Verification items for the finished model (mm, model axes). Face numbers are marked on the shaded views. A direction names the side the tool comes from. Coordinates: 2 decimals unless noted, no trailing zeros. Loops run counter-clockwise (first coordinate to the right, second up) from the corner with the lowest first, then second, coordinate; pieces in that order, holes last. Notation, with made-up numbers: (60.5, 18) -> (100.5, 18) arc R34 ccw to (100.5, 55) -> close; hole circle Ø5 at (-39.5, -15). An arc over 180 degrees is marked (long way). Answer as a JSON object with one key per item and string values. Group by question number.
Q1. Cross-section at B-B on z = -21.75. Record the boundary of the cut face in (x, y), and give its area (4 significant figures).
Q2. Cross-section at A-A on x = 0. Record the boundary of the cut face in (y, z), and give its area (3 significant figures).
Q3. Release check for a two-part mould opening along Z. For the marked faces 4 and 5 record: released by +Z, released by -Z, zero draft, split by the parting line, or undercut.
Q4. Cross-section at D-D on z = -4. Record the boundary of the cut face in (x, y), and give its area (3 significant figures).
Q5. Gauge pin test, flat ends, axial feed: pin 1 Ø1.5 at (y, z) = (3, 2.5) entering from +X; pin 2 Ø2 at (x, y) = (-1.5, 3.5) entering from -Z; pin 3 Ø1.5 at (x, y) = (1.5, 3) entering from +Z. Record the tip position at first contact, or that the pin passes through.
Q6. Cross-section at C-C on y = 3.7. Record the boundary of the cut face in (x, z).
Q7. Scan lines: L1, parallel to Z at x = 0, y = 4; L2, parallel to X at y = 4.25, z = -21.75; L3, parallel to Z at x = -1, y = 1.05. Record each from-to range of solid material in increasing order.
Q8. Set-up check for the marked faces 1, 2 and 3: record each of +Z, -Z, +X, -X, +Y, -Y from which the full face is reachable in a straight line by a thin tool's end or side.
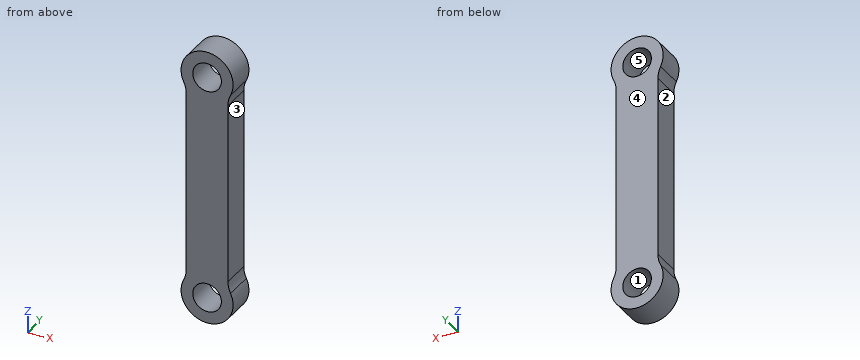
```python
from build123d import *

# Parameters (mm, degrees)
BOSS_EXTRUDE1_DEPTH = 5.5
SKETCH2_R           = 2.75
CUT_EXTRUDE2_DEPTH  = 6.5
SKETCH3_R           = 5
SKETCH3_R_2         = 2.75
BOSS_EXTRUDE2_DEPTH = 5.5
FILLET1_R           = 5


with BuildPart() as part:
    # Sketch1 → Boss-Extrude1 (new body)
    with BuildSketch(Plane(origin=(0, 0, 0), x_dir=(1, 0, 0), z_dir=(0, 1, 0))):
        with BuildLine():
            Line((-4, -21.75), (-4, 21.75))
            ThreePointArc((-4, 21.75), (0, 25.75), (4, 21.75))
            Line((4, 21.75), (4, -21.75))
            ThreePointArc((4, -21.75), (0, -25.75), (-4, -21.75))
        make_face()
    extrude(amount=BOSS_EXTRUDE1_DEPTH)

    # Sketch2 → Cut-Extrude2 (cut, through all)
    with BuildSketch(Plane(origin=(0, 5.5, 0), x_dir=(1, 0, 0), z_dir=(0, 1, 0))):
        with Locations((0, 21.75)):
            Circle(SKETCH2_R)
        with Locations((0, -21.75)):
            Circle(SKETCH2_R)
    extrude(amount=-CUT_EXTRUDE2_DEPTH, mode=Mode.SUBTRACT)

    # Sketch3 → Boss-Extrude2 (add)
    with BuildSketch(Plane(origin=(0, 5.5, 0), x_dir=(1, 0, 0), z_dir=(0, 1, 0))):
        with Locations((0, 21.75)):
            Circle(SKETCH3_R)
        with Locations((0, 21.75)):
            Circle(SKETCH3_R_2, mode=Mode.SUBTRACT)
        with Locations((0, -21.75)):
            Circle(SKETCH3_R)
        with Locations((0, -21.75)):
            Circle(SKETCH3_R_2, mode=Mode.SUBTRACT)
    extrude(amount=-BOSS_EXTRUDE2_DEPTH)

    # Fillet1
    fillet1_edges = [part.edges().sort_by_distance(p)[0] for p in [
        (-4, 2.75, -18.75),
        (4, 2.75, -18.75),
        (-4, 2.75, 18.75),
        (4, 2.75, 18.75),
    ]]
    fillet(fillet1_edges, radius=FILLET1_R)


solid = part.part
```
Computed values:
{
 "1": {"outline": "(-5, 0) -> (-2.75, 0) -> (-2.75, 5.5) -> (-5, 5.5) -> close; (2.75, 0) -> (5, 0) -> (5, 5.5) -> (2.75, 5.5) -> close", "area": "24.75 mm²"},
 "2": {"outline": "(0, -26.75) -> (5.5, -26.75) -> (5.5, -24.5) -> (0, -24.5) -> close; (0, -19) -> (5.5, -19) -> (5.5, 19) -> (0, 19) -> close; (0, 24.5) -> (5.5, 24.5) -> (5.5, 26.75) -> (0, 26.75) -> close", "area": "234 mm²"},
 "3": {"face 4": "zero draft", "face 5": "undercut"},
 "4": {"outline": "(-4, 0) -> (4, 0) -> (4, 5.5) -> (-4, 5.5) -> close", "area": "44.0 mm²"},
 "5": {"pin 1": "stops at x = 4", "pin 2": "stops at z = -26.72", "pin 3": "stops at z = 26.69"},
 "6": {"outline": "(-4.5, -19.57) arc R5 ccw (long way) to (4.5, -19.57) arc R5 cw to (4, -17.39) -> (4, 17.39) arc R5 cw to (4.5, 19.57) arc R5 ccw (long way) to (-4.5, 19.57) arc R5 cw to (-4, 17.39) -> (-4, -17.39) arc R5 cw to start; hole circle Ø5.5 at (0, -21.75); hole circle Ø5.5 at (0, 21.75)"},
 "7": {"L1": "z = -26.75 to -24.5, -19 to 19, 24.5 to 26.75", "L2": "x = -5 to -2.75, 2.75 to 5", "L3": "z = -26.65 to -24.31, -19.19 to 19.19, 24.31 to 26.65"},
 "8": {"face 1": "+Y, -Y", "face 2": "-X, +Y, -Y", "face 3": "+X, +Y, -Y"}
}
